Work out the finished part from the listing and answer in its coordinate system (mm). A direction names the side the tool comes from. Give positions to 0.01 mm unless a question says otherwise; leave off trailing zeros. Order: outer loops, then holes, each group sorted by start corner. A loop starts at its lowest first (then second) coordinate and runs counter-clockwise, first axis right, second up. Notation, with made-up numbers: (25.25, 80.25) -> (29.25, 80.25) arc R14 ccw to (29.25, 98.25) -> close; hole circle Ø4 at (-30, 2). An arc over 180 degrees is marked (long way). Answer as CSV lines item,"result". Start each with the question number.
1. A cutting plane is placed at D-D (y = 1.2). Give the vertices of the cut face in (x, z), then the cut area to 3 significant figures.
2. A cutting plane is placed at C-C (x = 9.5). Give the vertices of the cut face in (y, z).
3. For a pull along X with two mould halves and no side action, classify faces 3 (the flat face through (0, 1, 37.5)), 4 (the cylindrical face through (-34.287, 1.268, -59.248)), 5 (the flat face through (0, 1, 60)) as released by +X, released by -X, zero draft, split by the parting line, or undercut.
4. A cutting plane is placed at B-B (x = 0). Give the vertices of the cut face in (y, z), then the cut area to 3 significant figures.
5. A cutting plane is placed at A-A (z = 29). Give the vertices of the cut face in (x, y).
6. Find the intervals of material crossed by L1, parallel to Z at x = 6, y = 0.5; L2, parallel to X at y = 1.75, z = -50; L3, parallel to X at y = 0.5, z = -36, in increasing order.
7. For faces 1 (the flat face through (0, 0, -1)), 2 (the flat face through (16.25, 1, -30)), determine the directions among +Z, -Z, +X, -X, +Y, -Y from which every point of the face is accessible in a straight line to the end or side of a thin tool.
from build123d import *

# Parameters (mm, degrees)
CROQUIS1_W              = 70
CROQUIS1_H              = 120
SALIENTE_EXTRUIR1_DEPTH = 2.5
REDONDEO1_R             = 2.5
CROQUIS2_W              = 32.5
CROQUIS2_H              = 15
CORTAR_EXTRUIR1_DEPTH   = 70.507193872
CROQUIS3_R              = 2.5
CORTAR_EXTRUIR2_DEPTH   = 70.507193872


with BuildPart() as part:
    # Croquis1 → Saliente-Extruir1 (new body)
    with BuildSketch(Plane(origin=(0, 0, 0), x_dir=(1, 0, 0), z_dir=(0, 1, 0))):
        Rectangle(CROQUIS1_W, CROQUIS1_H)
    extrude(amount=SALIENTE_EXTRUIR1_DEPTH)

    # Redondeo1
    redondeo1_edges = [part.edges().sort_by_distance(p)[0] for p in [
        (35, 1.25, 60),
        (-35, 1.25, 60),
        (-35, 1.25, -60),
        (35, 1.25, -60),
    ]]
    fillet(redondeo1_edges, radius=REDONDEO1_R)

    # Croquis2 → Cortar-Extruir1 (cut, through all)
    with BuildSketch(Plane(origin=(0, 2.5, 0), x_dir=(1, 0, 0), z_dir=(0, 1, 0))):
        with Locations((0, 30)):
            Rectangle(CROQUIS2_W, CROQUIS2_H)
        with Locations((0, -30)):
            Rectangle(CROQUIS2_W, CROQUIS2_H)
    extrude(amount=-CORTAR_EXTRUIR1_DEPTH, mode=Mode.SUBTRACT)

    # Croquis3 → Cortar-Extruir2 (cut, through all)
    with BuildSketch(Plane(origin=(0, 2.5, 0), x_dir=(1, 0, 0), z_dir=(0, 1, 0))):
        with Locations(Location((0, 50, 0), (0, 0, 270))):
            Circle(CROQUIS3_R)
        with Locations(Location((0, -50, 0), (0, 0, 270))):
            Circle(CROQUIS3_R)
    extrude(amount=-CORTAR_EXTRUIR2_DEPTH, mode=Mode.SUBTRACT)


solid = part.part
Answer sheet:
1,outline,"(-35, -57.5) arc R2.5 ccw to (-32.5, -60) -> (32.5, -60) arc R2.5 ccw to (35, -57.5) -> (35, 57.5) arc R2.5 ccw to (32.5, 60) -> (-32.5, 60) arc R2.5 ccw to (-35, 57.5) -> close; hole (-16.25, -37.5) -> (16.25, -37.5) -> (16.25, -22.5) -> (-16.25, -22.5) -> close; hole (-16.25, 22.5) -> (16.25, 22.5) -> (16.25, 37.5) -> (-16.25, 37.5) -> close; hole circle Ø5 at (0, -50); hole circle Ø5 at (0, 50)"
1,area,"7,380 mm^2"
2,outline,"(0, -60) -> (2.5, -60) -> (2.5, -37.5) -> (0, -37.5) -> close; (0, -22.5) -> (2.5, -22.5) -> (2.5, 22.5) -> (0, 22.5) -> close; (0, 37.5) -> (2.5, 37.5) -> (2.5, 60) -> (0, 60) -> close"
3,face 3,"undercut"
3,face 4,"released by -X"
3,face 5,"zero draft"
4,outline,"(0, -60) -> (2.5, -60) -> (2.5, -52.5) -> (0, -52.5) -> close; (0, -47.5) -> (2.5, -47.5) -> (2.5, -37.5) -> (0, -37.5) -> close; (0, -22.5) -> (2.5, -22.5) -> (2.5, 22.5) -> (0, 22.5) -> close; (0, 37.5) -> (2.5, 37.5) -> (2.5, 47.5) -> (0, 47.5) -> close; (0, 52.5) -> (2.5, 52.5) -> (2.5, 60) -> (0, 60) -> close"
4,area,"200 mm^2"
5,outline,"(-35, 0) -> (-16.25, 0) -> (-16.25, 2.5) -> (-35, 2.5) -> close; (16.25, 0) -> (35, 0) -> (35, 2.5) -> (16.25, 2.5) -> close"
6,L1,"z = -60 to -37.5, -22.5 to 22.5, 37.5 to 60"
6,L2,"x = -35 to -2.5, 2.5 to 35"
6,L3,"x = -35 to -16.25, 16.25 to 35"
7,face 1,"+Z, -Z, +X, -X, -Y"
7,face 2,"+Y, -Y"
